Design review of the part built by this model. Coordinates are the model's own, in mm. A direction names the side the tool comes from. Coordinates: 2 decimals unless noted, no trailing zeros. Loops run counter-clockwise (first coordinate to the right, second up) from the corner with the lowest first, then second, coordinate; pieces in that order, holes last. Notation, with made-up numbers: (57, 50) -> (87, 50) arc R13 cw to (87, 64) -> close; hole circle Ø3 at (-1, 46.25). An arc over 180 degrees is marked (long way). Use one line per item in the form item = value. Start each with the question number.
1. Consider section A-A (z = -20). State the section outline as (x, y) points, then the cut area to 3 significant figures.
2. Consider section D-D (y = 2.45). State how many separate pieces and enclosed holes the cut face has, then the cut area to 3 significant figures.
3. The part is to be moulded in two halves that separate along X. For faces 1 (the face through (46.356, 1.479, -78.111)), 2 (the face through (46.267, 1.479, 12.448)), 3 (the face through (21, 0, -41)), say which applies: released by +X, released by -X, zero draft, split by the parting line, or undercut.
4. Consider section B-B (x = -1). State the section outline as (y, z) points, then the cut area to 3 significant figures.
5. Consider section C-C (x = 101.5). State the section outline as (y, z) points, then the cut area to 3 significant figures.
6. For pin 1 (1.5 mm diameter, centred on x = -109, y = 2, fed in from +Z); pin 2 (4 mm diameter, centred on x = 113.63, z = 65.95, fed in from +Y); pin 3 (0.9 mm diameter, centred on y = 1.5, z = -81.5, fed in from +X), all flat-tipped, find the tip position at first contact; note any pin that passes through.
7. Wall thickness on line 1 (X direction, y = 2.2, z = -91.5); line 2 (X direction, y = 1.25, z = -69); line 3 (X direction, y = 1.15, z = -45): over which ranges is each line inside the solid? List them lowest first. Write a range as from..to.
8. Machinability: for faces 4 (the face through (-38.579, 1.479, -77.595)), 5 (the face through (158.895, 1.479, 58.748)), which of the approach directions +Z, -Z, +X, -X, +Y, -Y give a long, thin tool a straight path to every point of the face, cutting with its end or side? Answer none if there is none.
from build123d import *

# Parameters (mm, degrees)
F0_R     = 0.875
F1_DEPTH = 1
F2_SCALE = 3


with BuildPart() as f1:
    # F0 (on Front) → F1 (new body)
    with BuildSketch(Plane.XZ):
        with BuildLine():
            Line((-9.5, -65.0096278997), (50, -65.0096278997))
            Line((50, -65.0096278997), (70.3501985279, -9.0979169629))
            ThreePointArc((70.3501985279, -9.0979169629), (70.0513622891, -8.4570605809), (70.6922186712, -8.1582243421))
            Line((70.6922186712, -8.1582243421), (73.9414100328, 0.7688555553))
            Line((73.9414100328, 0.7688555553), (43.9414100328, 6.0586649766))
            Line((43.9414100328, 6.0586649766), (40.6922186712, -2.8684149209))
            ThreePointArc((40.6922186712, -2.8684149209), (40.9910549099, -3.5092713029), (40.3501985279, -3.8081075417))
            Line((40.3501985279, -3.8081075417), (28.9937738537, -35.0096278997))
            Line((28.9937738537, -35.0096278997), (-9.5, -35.0096278997))
            ThreePointArc((-9.5, -35.0096278997), (-10, -35.5096278997), (-10.5, -35.0096278997))
            Line((-10.5, -35.0096278997), (-20, -35.0096278997))
            Line((-20, -35.0096278997), (-20, -65.0096278997))
            Line((-20, -65.0096278997), (-10.5, -65.0096278997))
            ThreePointArc((-10.5, -65.0096278997), (-10, -64.5096278997), (-9.5, -65.0096278997))
        make_face()
        with Locations((-15, -60.0096278997)):
            Circle(F0_R, mode=Mode.SUBTRACT)
        with Locations((-15, -50.0096278997)):
            Circle(F0_R, mode=Mode.SUBTRACT)
        with BuildLine():
            ThreePointArc((-1.4264235636, -54.7336339889), (-2.4617486132, -54.8014927777), (-3, -53.9144819446))
            Line((-3, -53.9144819446), (-3, -43.0096278997))
            ThreePointArc((-3, -43.0096278997), (-2.7071067812, -42.3025211185), (-2, -42.0096278997))
            Line((-2, -42.0096278997), (13.573745568, -42.0096278997))
            ThreePointArc((13.573745568, -42.0096278997), (14.5274625188, -42.7089221002), (14.1473220044, -43.828779944))
            Line((14.1473220044, -43.828779944), (-1.4264235636, -54.7336339889))
        make_face(mode=Mode.SUBTRACT)
        with BuildLine():
            ThreePointArc((39.7240060892, -56.4360514633), (39.7918648781, -57.4713765129), (38.9048540449, -58.0096278997))
            Line((38.9048540449, -58.0096278997), (9.2706946342, -58.0096278997))
            ThreePointArc((9.2706946342, -58.0096278997), (8.3169776835, -57.3103336992), (8.6971181979, -56.1904758554))
            Line((8.6971181979, -56.1904758554), (28.5819376277, -42.2669753947))
            ThreePointArc((28.5819376277, -42.2669753947), (29.3291622417, -42.101319686), (29.9746661083, -42.5125510026))
            Line((29.9746661083, -42.5125510026), (39.7240060892, -56.4360514633))
        make_face(mode=Mode.SUBTRACT)
        with Locations((-15, -40.0096278997)):
            Circle(F0_R, mode=Mode.SUBTRACT)
        with BuildLine():
            Line((57.3523945133, -24.3424591944), (47.2169150643, -52.1894601158))
            ThreePointArc((47.2169150643, -52.1894601158), (46.4077486357, -52.8388848339), (45.4580703992, -52.4210164089))
            Line((45.4580703992, -52.4210164089), (35.7087304184, -38.4975159482))
            ThreePointArc((35.7087304184, -38.4975159482), (35.5430747096, -37.7502913341), (35.9543060263, -37.1047874675))
            Line((35.9543060263, -37.1047874675), (55.8391254561, -23.1812870068))
            ThreePointArc((55.8391254561, -23.1812870068), (57.0214633215, -23.2070857108), (57.3523945133, -24.3424591944))
        make_face(mode=Mode.SUBTRACT)
        with BuildLine():
            ThreePointArc((42.3588515407, -24.0748542982), (41.1765136753, -24.0490555942), (40.8455824836, -22.9136821106))
            Line((40.8455824836, -22.9136821106), (44.8031451361, -12.0403680867))
            ThreePointArc((44.8031451361, -12.0403680867), (45.2428377569, -11.5163628263), (45.9164859345, -11.397580477))
            Line((45.9164859345, -11.397580477), (55.1599311689, -13.0274492665))
            ThreePointArc((55.1599311689, -13.0274492665), (55.9625789983, -13.7958174056), (55.5598594276, -14.8314090638))
            Line((55.5598594276, -14.8314090638), (42.3588515407, -24.0748542982))
        make_face(mode=Mode.SUBTRACT)
        with Locations((47.1289670212, 0.4194796176)):
            Circle(F0_R, mode=Mode.SUBTRACT)
        with Locations((67.2808894911, -3.133848027)):
            Circle(F0_R, mode=Mode.SUBTRACT)
        with Locations((57.2049282561, -1.3571842047)):
            Circle(F0_R, mode=Mode.SUBTRACT)
    extrude(amount=-F1_DEPTH)


with BuildPart() as f1_1:
    # F2: moved
    add(f1.part.scale(F2_SCALE).moved(Location((-57.9875477074, 0, 70.0192557993))))


solid = f1_1.part
Geometry check:
q1.outline = (34.46, 0) -> (80.29, 0) -> (80.29, 3) -> (34.46, 3) -> close; (107.89, 0) -> (130.23, 0) -> (130.23, 3) -> (107.89, 3) -> close
q1.area = 205 mm²
q2.separate_pieces = 1
q2.enclosed_holes = 10
q2.area = 24,200 mm²
q3.face_1 = undercut
q3.face_2 = released by -X
q3.face_3 = zero draft
q4.outline = (0, -125.01) -> (3, -125.01) -> (3, -104.01) -> (0, -104.01) -> close; (0, -76.92) -> (3, -76.92) -> (3, -35.01) -> (0, -35.01) -> close
q4.area = 189 mm²
q5.outline = (0, -98.94) -> (3, -98.94) -> (3, -37.54) -> (0, -37.54) -> close; (0, -5.15) -> (3, -5.15) -> (3, 20.49) -> (0, 20.49) -> close; (0, 31.99) -> (3, 31.99) -> (3, 83.32) -> (0, 83.32) -> close
q5.area = 415 mm²
q6.pin_1 = -35.01
q6.pin_2 = through
q6.pin_3 = 108.01
q7.line_1 = -117.99..-66.99, -58.44..-21.82, 55.73..104.21
q7.line_2 = -117.99..-66.99, -26.3..10.31, 39.98..65.61, 90.05..112.4
q7.line_3 = -117.99..48.87, 98.79..121.13
q8.face_4 = +Y, -Y
q8.face_5 = -Z, +X, +Y, -Y
